Read the model definition and answer for the solid it produces. Units are mm, in the model's axes. Face numbers are marked on the shaded views. A direction names the side the tool comes from. Coordinates: 2 decimals unless noted, no trailing zeros. Write each loop counter-clockwise with the first axis right and the second up, starting at its lowest first coordinate (ties: lowest second). Pieces come first, ordered by that corner, then holes. Notation, with made-up numbers: (-30.5, 32.25) - (-16.5, 32.25) arc R28 cw to (-16.5, 67.25) - close; hole circle Ø4 at (29, -26). An arc over 180 degrees is marked (long way). Use a Markdown table: item, result.
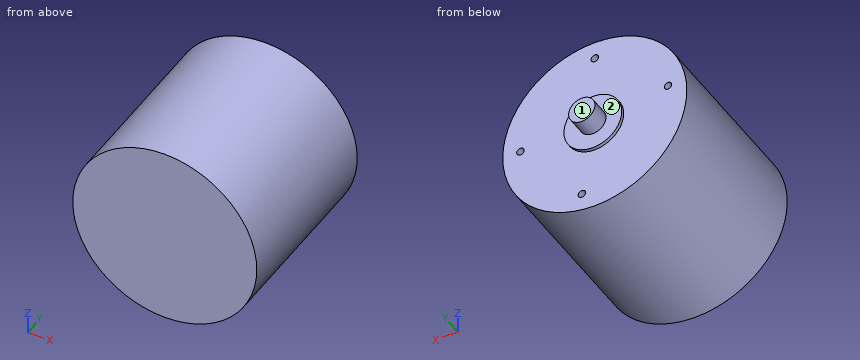
from build123d import *

# Parameters (mm, degrees)
F0_R     = 17.5
F1_DEPTH = 30
F2_R     = 38.5
F3_DEPTH = 4.5
F4_R     = 122.5
F5_DEPTH = 232
F6_R     = 5
F7_DEPTH = 25


with BuildPart() as f1:
    # F0 (on Front) → F1 (new body)
    with BuildSketch(Plane.XZ):
        Circle(F0_R)
    extrude(amount=-F1_DEPTH)

    # F2 (on Front) → F3 (join)
    with BuildSketch(Plane.XZ):
        Circle(F2_R)
    extrude(amount=-F3_DEPTH)

    # F4 (on Front) → F5 (join)
    with BuildSketch(Plane.XZ):
        Circle(F4_R)
    extrude(amount=F5_DEPTH)

    # F6 (on face) → F7 (cut)
    with BuildSketch(Plane(origin=(0, 0, 0), x_dir=(-1, 0, 0), z_dir=(0, 1, 0))):
        with Locations((-99, 0)):
            Circle(F6_R)
        with Locations((0, 99)):
            Circle(F6_R)
        with Locations((97.495968, 17.19117)):
            Circle(F6_R)
        with Locations((-17.19117, -97.495968)):
            Circle(F6_R)
    extrude(amount=-F7_DEPTH, mode=Mode.SUBTRACT)


solid = f1.part
(1) A cutting plane is placed at B-B, the plane x = 0. Write down the section's boundary in (y, z).
Report:
| item | result |
|---|---|
| outline | (-232, -122.5) - (0, -122.5) - (0, -38.5) - (4.5, -38.5) - (4.5, -17.5) - (30, -17.5) - (30, 17.5) - (4.5, 17.5) - (4.5, 38.5) - (0, 38.5) - (0, 94) - (-25, 94) - (-25, 104) - (0, 104) - (0, 122.5) - (-232, 122.5) - close |
(2) A cutting plane is placed at A-A, the plane z = 0. Write down the section's boundary in (x, y).
Report:
| item | result |
|---|---|
| outline | (-122.5, -232) - (122.5, -232) - (122.5, 0) - (104, 0) - (104, -25) - (94, -25) - (94, 0) - (38.5, 0) - (38.5, 4.5) - (17.5, 4.5) - (17.5, 30) - (-17.5, 30) - (-17.5, 4.5) - (-38.5, 4.5) - (-38.5, 0) - (-122.5, 0) - close |
(3) Each of these flat-tipped pins is pushed along its axis until it touches: P1, Ø10, axis at x = 87.5, z = 70, coming from the +Y side; P2, Ø6, axis at x = 99, z = 0, coming from the +Y side; P3, Ø10, axis at y = -199, z = 48, coming from the -X side. Where does it stop, or does it pass through?
Report:
| item | result |
|---|---|
| P1 | stops at y = 0 |
| P2 | stops at y = -25 |
| P3 | stops at x = -114.71 |
(4) For the marked faces 1 and 2, determine the directions among +Z, -Z, +X, -X, +Y, -Y from which every point of the face is accessible in a straight line to the end or side of a thin tool.
Report:
| item | result |
|---|---|
| face 1 | +Z, -Z, +X, -X, +Y |
| face 2 | +Y |
(5) A cutting plane is placed at C-C, the plane y = -141. Write down the section's boundary in (x, z), and give its area (3 significant figures).
Report:
| item | result |
|---|---|
| outline | circle Ø245 at (0, 0) |
| area | 47,100 mm² |
(6) A cutting plane is placed at D-D, the plane z = 99. Write down the section's boundary in (x, y).
Report:
| item | result |
|---|---|
| outline | (-72.15, -232) - (72.15, -232) - (72.15, 0) - (5, 0) - (5, -25) - (-5, -25) - (-5, 0) - (-72.15, 0) - close |
(7) Straight lines are drawn through the part: L1, parallel to Y at x = 78, z = 36.5; L2, parallel to Z at x = 99, y = -18.5; L3, parallel to X at y = -75, z = -68. For each, find the intervals that lie inside material, in ascending order.
Report:
| item | result |
|---|---|
| L1 | y = -232 to 0 |
| L2 | z = -72.15 to -5, 5 to 72.15 |
| L3 | x = -101.89 to 101.89 |
